Could you check a few things on this model? Use its own coordinates, in mm. Round coordinates to 2 decimals unless told otherwise and drop trailing zeros. Loops run counter-clockwise (first coordinate to the right, second up) from the corner with the lowest first, then second, coordinate; pieces in that order, holes last. Notation, with made-up numbers: (-22.5, 45.25) - (-3.5, 45.25) arc R19 cw to (-3.5, 71.25) - close; hole circle Ø11 at (72.5, 3). An arc over 180 degrees is marked (long way). Answer as CSV lines item,"result". Start each with the question number.
1) Suppose I cut it at B-B, the plane z = 68. Write out the boundary of the cut face in (x, y), then the cut area to 3 significant figures.
2) We'd pull the mould along X, two halves only. Please class faces 1 (the face through (144.618, 326.697, 37.567)), 2 (the face through (142.428, 324.285, 37.567)): pulls with the +X half, pulls with the -X half, needs draft (parallel to the pull), parting line crosses it, or undercut.
3) I'm going to push flat-ended pins straight in: pin 1 Ø8 at (x, z) = (303.5, 28) entering from -Y; pin 2 Ø10 at (x, z) = (-135, 50.5) entering from -Y; pin 3 Ø4 at (y, z) = (180.5, 27) entering from -X. Where does each tip first touch, or does it pass through?
4) Please list where these lines run through material, in increasing order: line 1 along X through (y, z) = (292.5, 42); line 2 along X through (y, z) = (298, 40); line 3 along X through (y, z) = (-14.5, 20.5).
Autodesk Inventor part; units mm, degrees
ref_plane "Work Plane3" through (383.5416, -39.2939, 0) normal (0.9993, -0.0363, 0) x (0.0363, 0.9993, 0)
ref_plane "Work Plane4" through (-271.6172, 233.6803, 0) normal (-0.7295, 0.684, 0) x (-0.684, -0.7295, 0)
ref_plane "YZ Plane" through (0, 0, 0) normal (1, 0, 0) x (0, 1, 0)
sketch "Sketch1" plane through (0, 0, 0) normal (0, 0, 1) x (1, 0, 0)
  arc A0 (380.5355, -38.0375) -> (-270.1768, 230.7579) centre (4.8231, -25.5444) ccw
  arc A1 (383.5416, -39.2939) -> (-271.6172, 233.6803) centre (4.8231, -25.5444) ccw
  line L0 (-271.6172, 233.6803) -> (-270.1768, 230.7579)
  line L1 (380.5355, -38.0375) -> (383.5416, -39.2939)
  point P0 (0, 0)
  dimension "d0" = 375.92
  dimension "d1" = 138.92
  dimension "d3" = 138.92
  dimension "d4" = 378.968
extrude "Extrusion1" add sketch "Sketch1" along normal blind 76.2
ref_plane "Work Plane3" through (383.5416, -39.2939, 0) normal (0.9993, -0.0363, 0) x (0.0363, 0.9993, 0)
ref_plane "Work Plane4" through (-271.6172, 233.6803, 0) normal (-0.7295, 0.684, 0) x (-0.684, -0.7295, 0)
sketch "Sketch2" plane through (383.5416, -39.2939, 0) normal (0.9993, -0.0363, 0) x (0.0363, 0.9993, 0)
  line L0 (249.0245, 76.2) -> (0, 76.2)
  line L1 (0, 0) -> (0, 76.2)
  line L2 (249.0245, 0) -> (0, 0)
  line L3 (249.0245, 0) -> (249.0245, 76.2)
  point P0 (25.3526, 0)
  point P1 (38.1, 57.15)
  point P2 (38.1, 38.1)
  point P3 (38.1, 19.05)
  dimension "d7" = 38.1
  dimension "d8" = 38.1
  dimension "d9" = 38.1
  dimension "d10" = 19.05
  dimension "d11" = 38.1
  dimension "d12" = 57.15
sketch "Sketch3" plane through (-271.6172, 233.6803, 0) normal (-0.7295, 0.684, 0) x (-0.684, -0.7295, 0)
  line L0 (0, 0) -> (0, 76.2)
  line L1 (-378.968, 0) -> (0, 0)
  point P0 (-15.3344, 0)
  point P1 (-38.1, 19.05)
  point P2 (-38.1, 38.1)
  point P3 (-38.1, 57.15)
  point P4 (-249.0245, 0)
  dimension "d13" = 38.1
  dimension "d14" = 38.1
  dimension "d15" = 38.1
  dimension "d16" = 19.05
  dimension "d17" = 38.1
  dimension "d18" = 57.15
hole "Hole1" at (-245.5557, 261.4726, 57.15) at (-245.5557, 261.4726, 38.1) at (-245.5557, 261.4726, 19.05) direction (0.7295, -0.684, 0) diameter 6.35 depth 25.4 tip angle 118
hole "Hole2" at (384.924, -1.219, 57.15) at (384.924, -1.219, 38.1) at (384.924, -1.219, 19.05) direction (-0.9993, 0.0363, 0) diameter 6.35 depth 25.4 tip angle 118
thread "Thread1"
thread "Thread2"
thread "Thread3"
thread "Thread4"
thread "Thread5"
thread "Thread6"
equation "\"d3\" = d1"
properties part number "curvedTrack"
Filled sheet:
1,outline,"(-271.62, 233.68) - (-270.18, 230.76) arc R375.92 cw to (380.54, -38.04) - (383.54, -39.29) arc R378.97 ccw to start"
1,area,"2,790 mm²"
2,face 1,"parting line crosses it"
2,face 2,"undercut"
3,pin 1,"y = 197.4"
3,pin 2,"y = 321.36"
3,pin 3,"x = 317.93"
4,line 1,"-201.25 to -195.59, 205.23 to 210.89"
4,line 2,"-192.5 to -186.58, 196.23 to 202.14"
4,line 3,"380.58 to 383.63"
